from build123d import *

# Parameters (mm, degrees)
F0_W     = 254
F0_H     = 50.8
F1_DEPTH = 609.6
F2_R     = 30.1625
F3_DEPTH = 107.192695


with BuildPart() as f1:
    # F0 (on Right) → F1 (new body)
    with BuildSketch(Plane.YZ):
        with Locations((-10.621817, -25.4)):
            Rectangle(F0_W, F0_H)
    extrude(amount=F1_DEPTH)

    # F2 (on Top) → F3 (cut)
    with BuildSketch(Plane.XY):
        with Locations((42.8625, -69.359317)):
            Circle(F2_R)
        with Locations((83.82, 48.115683)):
            Circle(F2_R)
        with Locations((129.54, -69.041817)):
            Circle(F2_R)
        with Locations((169.545, 48.115683)):
            Circle(F2_R)
        with Locations((215.265, -69.041817)):
            Circle(F2_R)
        with Locations((302.26, -69.041817)):
            Circle(F2_R)
        with BuildLine():
            ThreePointArc((388.63007, -38.561817), (367.301962, -90.052425), (418.79257, -68.724317))
            ThreePointArc((418.79257, -68.724317), (409.958178, -47.396209), (388.63007, -38.561817))
        make_face()
        with BuildLine():
            ThreePointArc((505.143344, -68.724317), (496.308952, -47.396209), (474.980844, -38.561817))
            ThreePointArc((474.980844, -38.561817), (453.652735, -90.052425), (505.143344, -68.724317))
        make_face()
        with Locations((341.63, 48.115683)):
            Circle(F2_R)
        with Locations((429.26, 47.798183)):
            Circle(F2_R)
        with Locations((515.62, 47.798183)):
            Circle(F2_R)
        with Locations((561.6575, -69.041817)):
            Circle(F2_R)
    extrude(amount=-F3_DEPTH, mode=Mode.SUBTRACT)


solid = f1.part
Geometry check sheet. Reference: the model listing, model coordinates, mm. Round coordinates to 2 decimals unless told otherwise and drop trailing zeros. Loops run counter-clockwise (first coordinate to the right, second up) from the corner with the lowest first, then second, coordinate; pieces in that order, holes last. Notation, with made-up numbers: (-27.5, 59.5) -> (21.5, 59.5) arc R25 ccw to (21.5, 87.5) -> close; hole circle Ø1 at (-38, 73.25). An arc over 180 degrees is marked (long way). Answer as a JSON object with one key per item and string values. Group by question number.
Item 1: Cross-section at B-B, the plane y = 68.5. Record the cut outline in (x, z), plus the area to 3 significant figures.
Item 2: Cross-section at C-C, the plane z = -24.5. Count the separate pieces of the cut face and the enclosed holes in it, plus the area to 3 significant figures.
Item 3: Cross-section at D-D, the plane x = 166.5. Record the cut outline in (y, z).
Item 4: Thickness scan on line 1 along X through (y, z) = (46.5, -34); line 2 along Y through (x, z) = (515.62, -32); line 3 along X through (y, z) = (51, -12). Record the ranges inside material, lowest first.
Item 5: Cross-section at A-A, the plane x = 429.26. Record the cut outline in (y, z), plus the area to 3 significant figures.
Item 6: Depth check by flat-ended pin: pin 1 Ø10 at (x, y) = (113, 41.5) entering from +Z. Enter the tip coordinate at first touch or a pass-through.
Item 7: Release check for a two-part mould opening along X. For faces 1 (the face through (370.4, 57.18, -25.04)), 2 (the face through (0, -12, -25)), 3 (the face through (301, -12, 0)), 4 (the face through (139.41, 49.44, -25.04)) record: pulls with the +X half, pulls with the -X half, needs draft (parallel to the pull), parting line crosses it, or undercut.
Determined:
{
 "1": {"outline": "(0, -50.8) -> (61.59, -50.8) -> (61.59, 0) -> (0, 0) -> close; (106.05, -50.8) -> (147.31, -50.8) -> (147.31, 0) -> (106.05, 0) -> close; (191.78, -50.8) -> (319.4, -50.8) -> (319.4, 0) -> (191.78, 0) -> close; (363.86, -50.8) -> (407.32, -50.8) -> (407.32, 0) -> (363.86, 0) -> close; (451.2, -50.8) -> (493.68, -50.8) -> (493.68, 0) -> (451.2, 0) -> close; (537.56, -50.8) -> (609.6, -50.8) -> (609.6, 0) -> (537.56, 0) -> close", "area": "19,700 mm²"},
 "2": {"separate pieces": "1", "enclosed holes": "12", "area": "121,000 mm²"},
 "3": {"outline": "(-137.62, -50.8) -> (18.11, -50.8) -> (18.11, 0) -> (-137.62, 0) -> close; (78.12, -50.8) -> (116.38, -50.8) -> (116.38, 0) -> (78.12, 0) -> close"},
 "4": {"line 1": "x = 0 to 53.7, 113.94 to 139.43, 199.66 to 311.51, 371.75 to 399.13, 459.39 to 485.49, 545.75 to 609.6", "line 2": "y = -137.62 to 17.64, 77.96 to 116.38", "line 3": "x = 0 to 53.8, 113.84 to 139.52, 199.57 to 311.61, 371.65 to 399.27, 459.25 to 485.63, 545.61 to 609.6"},
 "5": {"outline": "(-137.62, -50.8) -> (17.64, -50.8) -> (17.64, 0) -> (-137.62, 0) -> close; (77.96, -50.8) -> (116.38, -50.8) -> (116.38, 0) -> (77.96, 0) -> close", "area": "9,840 mm²"},
 "6": {"pin 1": "stops at z = 0"},
 "7": {"face 1": "undercut", "face 2": "pulls with the -X half", "face 3": "needs draft", "face 4": "undercut"}
}
